```python
from build123d import *

# Parameters (mm, degrees)
BOSS_EXTRUDE1_DEPTH = 5
SKETCH2_W           = 10
SKETCH2_H           = 8
BOSS_EXTRUDE2_DEPTH = 2
BOSS_EXTRUDE3_DEPTH = 20.25
SKETCH4_R           = 1.25
SKETCH4_R_2         = 1.5
CUT_EXTRUDE1_DEPTH  = 59.259119458
SKETCH6_W           = 4.4
SKETCH6_H           = 2.75
BOSS_EXTRUDE4_DEPTH = 6.25
SKETCH7_W           = 20
SKETCH7_H           = 10
BOSS_EXTRUDE5_DEPTH = 15
CUT_EXTRUDE2_DEPTH  = 6
SKETCH9_R           = 4
CUT_EXTRUDE3_DEPTH  = 58.048772993
SKETCH10_W          = 3
SKETCH10_H          = 5
BOSS_EXTRUDE6_DEPTH = 4


with BuildPart() as part:
    # Sketch1 → Boss-Extrude1 (new body)
    with BuildSketch(Plane.XY):
        Polygon((0, 0), (44, 0), (44, 10), (32, 10), (32, 28), (12, 28), (12, 10), (0, 10), align=None)
    extrude(amount=BOSS_EXTRUDE1_DEPTH)

    # Sketch2 → Boss-Extrude2 (add)
    with BuildSketch(Plane.XY.offset(5)):
        with Locations((39, 4)):
            Rectangle(SKETCH2_W, SKETCH2_H)
        with Locations((5, 4)):
            Rectangle(SKETCH2_W, SKETCH2_H)
    extrude(amount=BOSS_EXTRUDE2_DEPTH)

    # Sketch3 → Boss-Extrude3 (add)
    with BuildSketch(Plane.XY.offset(7)):
        Polygon((37.6, 0), (43, 0), (43, 4), (42, 4), (42, 1.25), (37.6, 1.25), align=None)
        Polygon((1, 0), (6.4, 0), (6.4, 1.25), (2, 1.25), (2, 4), (1, 4), align=None)
    extrude(amount=BOSS_EXTRUDE3_DEPTH)

    # Sketch4 → Cut-Extrude1 (cut, through all)
    with BuildSketch(Plane(origin=(0, 1.25, 0), x_dir=(1, 0, 0), z_dir=(0, 1, 0))):
        with Locations(Location((40, -20.75, 0), (0, 0, 180))):
            Circle(SKETCH4_R)
        with Locations(Location((40, -24.25, 0), (0, 0, 180))):
            Circle(SKETCH4_R_2)
        with Locations(Location((4, -24.25, 0), (0, 0, 180))):
            Circle(SKETCH4_R_2)
        with Locations(Location((4, -17.25, 0), (0, 0, 180))):
            Circle(SKETCH4_R_2)
        with Locations(Location((4, -20.75, 0), (0, 0, 180))):
            Circle(SKETCH4_R)
        with Locations(Location((40, -17.25, 0), (0, 0, 180))):
            Circle(SKETCH4_R_2)
    extrude(amount=-CUT_EXTRUDE1_DEPTH, mode=Mode.SUBTRACT)

    # Sketch6 → Boss-Extrude4 (add)
    with BuildSketch(Plane.XY.offset(7)):
        with Locations((4.2, 2.625)):
            Rectangle(SKETCH6_W, SKETCH6_H)
        with Locations((39.8, 2.625)):
            Rectangle(SKETCH6_W, SKETCH6_H)
    extrude(amount=BOSS_EXTRUDE4_DEPTH)

    # Sketch7 → Boss-Extrude5 (add)
    with BuildSketch(Plane.XY.offset(5)):
        with Locations((22, 23)):
            Rectangle(SKETCH7_W, SKETCH7_H)
    extrude(amount=BOSS_EXTRUDE5_DEPTH)

    # Sketch8 → Cut-Extrude2 (cut)
    with BuildSketch(Plane.XZ.offset(-18)):
        Polygon((28.495190528, 12.5), (25.247595264, 18.125), (18.752404736, 18.125), (15.504809472, 12.5), (18.752404736, 6.875), (25.247595264, 6.875), align=None)
    extrude(amount=-CUT_EXTRUDE2_DEPTH, mode=Mode.SUBTRACT)

    # Sketch9 → Cut-Extrude3 (cut, through all)
    with BuildSketch(Plane.XZ.offset(-24)):
        with Locations(Location((22, 12.5, 0), (0, 0, 270))):
            Circle(SKETCH9_R)
    extrude(amount=-CUT_EXTRUDE3_DEPTH, mode=Mode.SUBTRACT)

    # Sketch10 → Boss-Extrude6 (add)
    with BuildSketch(Plane(origin=(0, 28, 0), x_dir=(1, 0, 0), z_dir=(0, 1, 0))):
        with Locations((30.5, -2.5)):
            Rectangle(SKETCH10_W, SKETCH10_H)
        with Locations((30.5, -17.5)):
            Rectangle(SKETCH10_W, SKETCH10_H)
        with Locations((13.5, -2.5)):
            Rectangle(SKETCH10_W, SKETCH10_H)
        with Locations((13.5, -17.5)):
            Rectangle(SKETCH10_W, SKETCH10_H)
    extrude(amount=BOSS_EXTRUDE6_DEPTH)


solid = part.part
```
Verification items for the finished model (mm, model axes). A direction names the side the tool comes from. Coordinates: 2 decimals unless noted, no trailing zeros. Write each loop counter-clockwise with the first axis right and the second up, starting at its lowest first coordinate (ties: lowest second). Pieces come first, ordered by that corner, then holes. Notation, with made-up numbers: (57, 17) - (95, 17) arc R25 cw to (95, 36) - close; hole circle Ø6 at (4.5, 59.5). An arc over 180 degrees is marked (long way). One line per question, with ' | ' between items. Start each with the question number.
1. Section check A-A (z = 24.25). Enter the section's corners in (x, y), plus the area to 3 significant figures.
2. Section check D-D (x = 40). Enter the section's corners in (y, z), plus the area to 3 significant figures.
3. Access from +Z, -Z, +X, -X, +Y, -Y to the whole of each face (thin tool, end or side, straight path). Record for faces 1 (the flat face through (13, 30, 15)), 2 (the flat face through (43, 2, 17)), 3 (the flat face through (4, 3, 13.25)).
4. Section check B-B (x = 22). Enter the section's corners in (y, z) (3 decimals), plus the area to 4 significant figures.
5. Material ranges on line 1 along Z through (x, y) = (4, 1.05); line 2 along X through (y, z) = (25, 12.5); line 3 along X through (y, z) = (30, 19.5), recorded low to high.
6. Gauge pin test, flat ends, axial feed: P1, Ø1.5, axis at x = 14, y = 29, coming from the -Z side; P2, Ø3, axis at y = 1.5, z = 18, coming from the -X side; P3, Ø2, axis at y = 3.5, z = 23, coming from the +X side; P4, Ø14.5, axis at x = 25, y = 4.5, coming from the +Z side. Record the tip position at first contact, or that the pin passes through.
7. Draft check along X on faces 4 (the flat face through (0, 5, 3)), 5 (the flat face through (10, 4, 6)), 6 (the flat face through (6, 10, 2)). Enter one of: released by +X, released by -X, zero draft, split by the parting line, or undercut.
8. Section check C-C (z = 17.25). Count the separate pieces of the cut face and the enclosed holes in it, plus the area to 3 significant figures.
Computed values:
1) outline: (1, 0) - (2.5, 0) - (2.5, 1.25) - (2, 1.25) - (2, 4) - (1, 4) - close; (5.5, 0) - (6.4, 0) - (6.4, 1.25) - (5.5, 1.25) - close; (37.6, 0) - (38.5, 0) - (38.5, 1.25) - (37.6, 1.25) - close; (41.5, 0) - (43, 0) - (43, 4) - (42, 4) - (42, 1.25) - (41.5, 1.25) - close | area: 11.5 mm²
2) outline: (0, 0) - (10, 0) - (10, 5) - (8, 5) - (8, 7) - (4, 7) - (4, 13.25) - (1.25, 13.25) - (1.25, 15.75) - (0, 15.75) - close; (0, 18.75) - (1.25, 18.75) - (1.25, 19.5) - (0, 19.5) - close; (0, 22) - (1.25, 22) - (1.25, 22.75) - (0, 22.75) - close; (0, 25.75) - (1.25, 25.75) - (1.25, 27.25) - (0, 27.25) - close | area: 97.9 mm²
3) face 1: +X, -X, +Y | face 2: +Z, +X, +Y, -Y | face 3: +Z, +Y
4) outline: (0, 0) - (28, 0) - (28, 8.5) - (24, 8.5) - (24, 6.875) - (18, 6.875) - (18, 5) - (0, 5) - close; (18, 18.125) - (24, 18.125) - (24, 16.5) - (28, 16.5) - (28, 20) - (18, 20) - close | area: 190.5 mm²
5) line 1: 0 to 15.75, 18.75 to 19.5, 22 to 22.75, 25.75 to 27.25 | line 2: 12 to 18, 26 to 32 | line 3: 12 to 15, 29 to 32
6) P1: z = 0 | P2: x = 1 | P3: x = 43 | P4: z = 5
7) face 4: released by -X | face 5: undercut | face 6: zero draft
8) separate pieces: 5 | enclosed holes: 0 | area: 190 mm²
